Part model, mm, in its own coordinate system. Face numbers are marked on the shaded views. A direction names the side the tool comes from. Round coordinates to 2 decimals unless told otherwise and drop trailing zeros. Write each loop counter-clockwise with the first axis right and the second up, starting at its lowest first coordinate (ties: lowest second). Pieces come first, ordered by that corner, then holes. Notation, with made-up numbers: (66, 70) -> (92, 70) arc R32 cw to (92, 102) -> close; hole circle Ø1 at (36, 31.25). An arc over 180 degrees is marked (long way). Return JSON: item names as keys, results as strings. Group by question number.
(1) Tool access for the marked faces 1, 2, 3 and 4: list every direction of +Z, -Z, +X, -X, +Y, -Y with a clear straight run to the whole face (end or side of a thin tool).
(2) Saw through at C-C (z = 14). List the corners of the cut face in (x, y), plus the area to 3 significant figures.
(3) Saw through at D-D (y = -14). List the corners of the cut face in (x, z).
(4) Drop flat-ended pins along their axis: pin 1 Ø10 at (y, z) = (11.5, 18) entering from -X; pin 2 Ø5 at (y, z) = (6, 13) entering from +X; pin 3 Ø7 at (y, z) = (3.5, 20) entering from +X. Give the stop position or say it passes through.
(5) Saw through at B-B (x = 0). List the corners of the cut face in (y, z).
(6) Saw through at A-A (z = 2). List the corners of the cut face in (x, y), plus the area to 3 significant figures.
(7) Drill centre lines: L1, parallel to Y at x = 0, z = 3.25; L2, parallel to X at y = -6, z = 15; L3, parallel to Z at x = 4.5, y = -9.5. Where is each one in solid material? Low to high. Write a range as from..to.
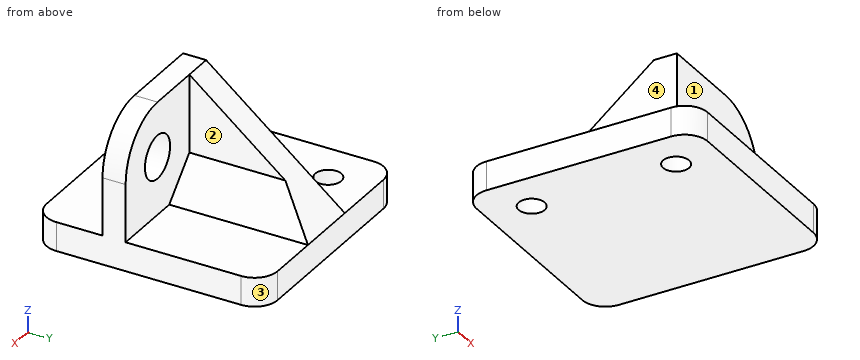
from build123d import *

# Parameters (mm, degrees)
SKETCH1_W           = 39.5
SKETCH1_H           = 40
SKETCH1_R           = 2.25
BOSS_EXTRUDE1_DEPTH = 5
BOSS_EXTRUDE2_START = -12
SKETCH2_R           = 3.75
BOSS_EXTRUDE2_DEPTH = 4
BOSS_EXTRUDE3_DEPTH = 5
FILLET1_R           = 4
CHAMFER2_SIZE       = 6


with BuildPart() as part:
    # Sketch1 → Boss-Extrude1 (new body)
    with BuildSketch(Plane.XY):
        with Locations((12.25, 0)):
            Rectangle(SKETCH1_W, SKETCH1_H)
        with Locations((0, 12.5)):
            Circle(SKETCH1_R, mode=Mode.SUBTRACT)
        with Locations((0, -12.5)):
            Circle(SKETCH1_R, mode=Mode.SUBTRACT)
    extrude(amount=BOSS_EXTRUDE1_DEPTH)

    # Sketch2 → Boss-Extrude2 (add)
    with BuildSketch(Plane.XZ.offset(20).offset(BOSS_EXTRUDE2_START)):
        with BuildLine():
            Line((32, 5), (13, 5))
            Line((13, 5), (13, 24.5))
            Line((13, 24.5), (22.5, 24.5))
            ThreePointArc((22.5, 24.5), (29.217514421, 21.717514421), (32, 15))
            Line((32, 15), (32, 5))
        make_face()
        with Locations(Location((22.5, 15, 0), (0, 0, 270))):
            Circle(SKETCH2_R, mode=Mode.SUBTRACT)
    extrude(amount=-BOSS_EXTRUDE2_DEPTH)

    # Sketch3 → Boss-Extrude3 (add)
    with BuildSketch(Plane.ZY.offset(-13)):
        Polygon((24.5, -4), (5, 20), (5, -4), (5, -8), (24.5, -8), align=None)
    extrude(amount=BOSS_EXTRUDE3_DEPTH)

    # Fillet1
    fillet1_edges = [part.edges().sort_by_distance(p)[0] for p in [
        (32, 20, 2.5),
        (-7.5, -20, 2.5),
        (-7.5, 20, 2.5),
        (32, -20, 2.5),
    ]]
    fillet(fillet1_edges, radius=FILLET1_R)

    # Chamfer2
    chamfer2_edges = [part.edges().sort_by_distance(p)[0] for p in [
        (13, 8, 5),
    ]]
    chamfer(chamfer2_edges, length=CHAMFER2_SIZE)


solid = part.part
Computed values:
{
 "1": {"face 1": "+Z, +X, -X, -Y", "face 2": "+Z, +X, +Y", "face 3": "+Z, -Z, +X, +Y", "face 4": "+Z, -X, +Y, -Y"},
 "2": {"outline": "(8, -8) -> (18.89, -8) -> (18.89, -4) -> (13, -4) -> (13, 8.92) -> (8, 8.92) -> close; (26.11, -8) -> (32, -8) -> (32, -4) -> (26.11, -4) -> close", "area": "132 mm2"},
 "3": {"outline": "(-7.5, 0) -> (-1.68, 0) -> (-1.68, 5) -> (-7.5, 5) -> close; (1.68, 0) -> (32, 0) -> (32, 5) -> (1.68, 5) -> close"},
 "4": {"pin 1": "x = 8", "pin 2": "x = 13.5", "pin 3": "x = 13"},
 "5": {"outline": "(-20, 0) -> (-14.75, 0) -> (-14.75, 5) -> (-20, 5) -> close; (-10.25, 0) -> (10.25, 0) -> (10.25, 5) -> (-10.25, 5) -> close; (14.75, 0) -> (20, 0) -> (20, 5) -> (14.75, 5) -> close"},
 "6": {"outline": "(-7.5, -16) arc R4 ccw to (-3.5, -20) -> (28, -20) arc R4 ccw to (32, -16) -> (32, 16) arc R4 ccw to (28, 20) -> (-3.5, 20) arc R4 ccw to (-7.5, 16) -> close; hole circle Ø4.5 at (0, -12.5); hole circle Ø4.5 at (0, 12.5)", "area": "1,530 mm2"},
 "7": {"L1": "-20..-14.75, -10.25..10.25, 14.75..20", "L2": "8..18.75, 26.25..32", "L3": "0..5"}
}
